```python
from build123d import *

# Parameters (mm, degrees)
F0_W     = 550
F0_H     = 550
F1_DEPTH = 6
F2_W     = 300
F2_H     = 300
F3_DEPTH = 6
F4_R     = 1.5
F4_R_2   = 10
F4_R_3   = 11
F4_R_4   = 2
F5_DEPTH = 25


with BuildPart() as f1:
    # F0 (on Top) → F1 (new body)
    with BuildSketch(Plane.XY):
        Rectangle(F0_W, F0_H)
    extrude(amount=F1_DEPTH)

    # F2 (on face) → F3 (cut, through all)
    with BuildSketch(Plane.XY.offset(6)):
        Rectangle(F2_W, F2_H)
    extrude(amount=-F3_DEPTH, mode=Mode.SUBTRACT)

    # F4 (on face) + F0 (on Top) → F5 (cut)
    with BuildSketch(Plane.XY.offset(6)):
        with Locations((-179, 253)):
            Circle(F4_R)
        with Locations((-210, 253)):
            Circle(F4_R)
        with Locations((-210, 222)):
            Circle(F4_R)
        with Locations((-179, 222)):
            Circle(F4_R)
        with Locations((-194.5, 237.5)):
            Circle(F4_R_2)
        with Locations((210, 253)):
            Circle(F4_R)
        with Locations((179, 253)):
            Circle(F4_R)
        with Locations((179, 222)):
            Circle(F4_R)
        with Locations((210, 222)):
            Circle(F4_R)
        with Locations((194.5, 237.5)):
            Circle(F4_R_2)
        with Locations((15.5, 253)):
            Circle(F4_R)
        with Locations((-15.5, 253)):
            Circle(F4_R)
        with Locations((-15.5, 222)):
            Circle(F4_R)
        with Locations((15.5, 222)):
            Circle(F4_R)
        with Locations((0, 237.5)):
            Circle(F4_R_2)
        with Locations((-177.5, -222)):
            Circle(F4_R)
        with Locations((-208.5, -222)):
            Circle(F4_R)
        with Locations((-208.5, -253)):
            Circle(F4_R)
        with Locations((-177.5, -253)):
            Circle(F4_R)
        with Locations((-193, -237.5)):
            Circle(F4_R_3)
        with Locations((210, -222)):
            Circle(F4_R)
        with Locations((179, -222)):
            Circle(F4_R)
        with Locations((179, -253)):
            Circle(F4_R)
        with Locations((210, -253)):
            Circle(F4_R)
        with Locations((194.5, -237.5)):
            Circle(F4_R_2)
        with Locations((15.5, -220.5)):
            Circle(F4_R)
        with Locations((-15.5, -220.5)):
            Circle(F4_R)
        with Locations((-15.5, -251.5)):
            Circle(F4_R)
        with Locations((15.5, -251.5)):
            Circle(F4_R)
        with Locations((0, -236)):
            Circle(F4_R_2)
        with Locations((-236, 193)):
            Circle(F4_R_4)
        with Locations((-204, 193)):
            Circle(F4_R_4)
        with Locations((-236, -193)):
            Circle(F4_R_4)
        with Locations((-204, -193)):
            Circle(F4_R_4)
        with Locations((236, -193)):
            Circle(F4_R_4)
        with Locations((204, -193)):
            Circle(F4_R_4)
        with Locations((204, 193)):
            Circle(F4_R_4)
        with Locations((236, 193)):
            Circle(F4_R_4)
    with BuildSketch(Plane.XY):
        Rectangle(F0_W, F0_H)
    extrude(amount=-F5_DEPTH, mode=Mode.SUBTRACT)


solid = f1.part
```
CAD build for the part. Positions are in the model's coordinates, mm. Coordinates: 2 decimals unless noted, no trailing zeros. Order: outer loops, then holes, each group sorted by start corner. A loop starts at its lowest first (then second) coordinate and runs counter-clockwise, first axis right, second up. Notation, with made-up numbers: (1, 65.25) -> (55, 65.25) arc R13 cw to (55, 78.25) -> close; hole circle Ø11 at (74, 55). An arc over 180 degrees is marked (long way). Use one line per item in the form item = value. Start each with the question number.
1) Band-saw the part on B-B on x = 194.5. Give the cut face in (y, z).
2) Drill centre lines: L1, parallel to X at y = 67, z = 4; L2, parallel to X at y = -193, z = 1.5. Where is each one in solid material? Low to high. Write a range as [from, to].
3) Drop a flat-ended pin along its axis: pin 1 (3 mm diameter, centred on x = 204, y = 193, fed in from +Z). Give the stop position or say it passes through.
4) Band-saw the part on D-D on z = 1.05. State how many separate pieces and enclosed holes the cut face has, then the cut area to 3 significant figures.
5) Band-saw the part on A-A on y = -5. Give the cut face in (x, z).
6) Pull direction Y, two halves, no side cores. Call faces 1 (the cylindrical face through (-201.11, -230.07, 3.04)), 2 (the flat face through (-4, 187, 6)): +Y half, -Y half, draft (parallel to the pull), parting line (faces both ways), or undercut.
Entries:
q1.outline = (-275, 0) -> (-247.5, 0) -> (-247.5, 6) -> (-275, 6) -> close; (-227.5, 0) -> (227.5, 0) -> (227.5, 6) -> (-227.5, 6) -> close; (247.5, 0) -> (275, 0) -> (275, 6) -> (247.5, 6) -> close
q2.L1 = [-275, -150], [150, 275]
q2.L2 = [-275, -238], [-234, -206], [-202, 202], [206, 234], [238, 275]
q3.pin_1 = through
q4.separate_pieces = 1
q4.enclosed_holes = 39
q4.area = 210,000 mm2
q5.outline = (-275, 0) -> (-150, 0) -> (-150, 6) -> (-275, 6) -> close; (150, 0) -> (275, 0) -> (275, 6) -> (150, 6) -> close
q6.face_1 = undercut
q6.face_2 = draft
